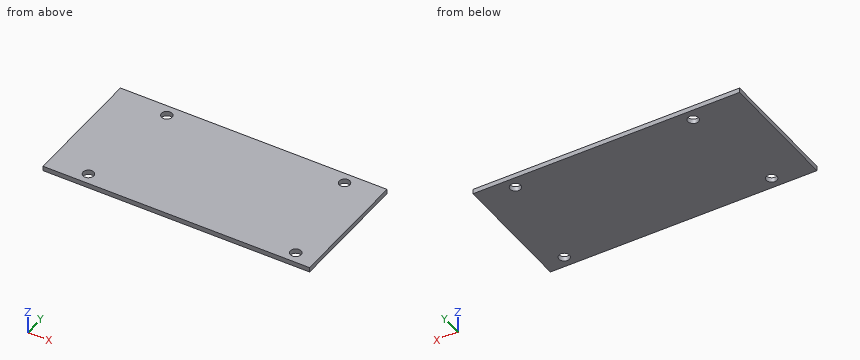
```python
from build123d import *

# Parameters (mm, degrees)
F0_W     = 90
F0_H     = 42.62
F1_DEPTH = 1.6
F2_D     = 3.6


with BuildPart() as f1:
    # F0 (on Top) → F1 (new body)
    with BuildSketch(Plane.XY):
        with Locations((45, 21.31)):
            Rectangle(F0_W, F0_H)
    extrude(amount=F1_DEPTH)

    # F2 (through all)
    with Locations(Plane(origin=(0, 0, 0), x_dir=(1, 0, 0), z_dir=(0, 0, -1))):
        with Locations((18, -38.81), (13, -3.81), (78, -38.81), (83, -3.81)):
            Hole(F2_D / 2)


solid = f1.part
```
Geometry check sheet. Reference: the model listing, model coordinates, mm. Coordinates: 2 decimals unless noted, no trailing zeros. Loops run counter-clockwise (first coordinate to the right, second up) from the corner with the lowest first, then second, coordinate; pieces in that order, holes last.
Item 1: Sectioned sample at B-B, the plane y = 3.81. Record the boundary of the cut face in (x, z).
Item 2: Go/stop test with a flat-tipped pin: pin 1 Ø6 at (x, y) = (78, 38.81) entering from -Z. Record where the tip stops, or that it passes through.
Item 3: Thickness scan on line 1 (X direction, y = 38.81, z = 0.6); line 2 (Y direction, x = 18, z = 1.55); line 3 (Y direction, x = 83, z = 0.6). Record the ranges inside material, lowest first.
Item 4: Sectioned sample at C-C, the plane y = 38. Record the boundary of the cut face in (x, z), then the cut area to 3 significant figures.
Item 5: Sectioned sample at A-A, the plane x = 78. Record the boundary of the cut face in (y, z).
Check result:
1. outline: (0, 0) - (11.2, 0) - (11.2, 1.6) - (0, 1.6) - close; (14.8, 0) - (81.2, 0) - (81.2, 1.6) - (14.8, 1.6) - close; (84.8, 0) - (90, 0) - (90, 1.6) - (84.8, 1.6) - close
2. pin 1: stops at z = 0
3. line 1: x = 0 to 16.2, 19.8 to 76.2, 79.8 to 90
3. line 2: y = 0 to 37.01, 40.61 to 42.62
3. line 3: y = 0 to 2.01, 5.61 to 42.62
4. outline: (0, 0) - (16.39, 0) - (16.39, 1.6) - (0, 1.6) - close; (19.61, 0) - (76.39, 0) - (76.39, 1.6) - (19.61, 1.6) - close; (79.61, 0) - (90, 0) - (90, 1.6) - (79.61, 1.6) - close
4. area: 134 mm2
5. outline: (0, 0) - (37.01, 0) - (37.01, 1.6) - (0, 1.6) - close; (40.61, 0) - (42.62, 0) - (42.62, 1.6) - (40.61, 1.6) - close
